Read the model definition and answer for the solid it produces. Units are mm, in the model's axes. A direction names the side the tool comes from. Coordinates: 2 decimals unless noted, no trailing zeros. Write each loop counter-clockwise with the first axis right and the second up, starting at its lowest first coordinate (ties: lowest second). Pieces come first, ordered by that corner, then holes.
(1) Section C-C on z = 3.25 is taken. Write down the section's boundary in (x, y), then the cut area to 3 significant figures.
(2) Which of the six approach directions +Z, -Z, +X, -X, +Y, -Y give full straight-line access (tool end or side, diameter ignored) to faces 4 (the flat face through (2, 0.5, -2)), 5 (the flat face through (7, 0, 10)), 6 (the cylindrical face through (-6.9, 6.95, 10.89))?
(3) The mould has two halves that part along X. Classify faces 1 (the flat face through (-0.598, 4.048, 7.732)), 2 (the cylindrical face through (6.93, 0.25, -4.4)), 3 (the cylindrical face through (-1.952, 0.246, -0.434)): +X half, -X half, draft (parallel to the pull), parting line (faces both ways), or undercut.
(4) Section B-B on z = 0 is taken. Write down the section's boundary in (x, y), then the cut area to 3 significant figures.
(5) Section A-A on x = 0 is taken. Write down the section's boundary in (y, z), then the cut area to 3 significant figures.
(6) Find the intervals of material crossed by probe 1 along X at (y, z) = (0.15, 0); probe 2 along Y at (x, z) = (2, 2.25); probe 3 along X at (y, z) = (4.75, 12.75), in increasing order.
(7) Section D-D on x = 1.5 is taken. Write down the section's boundary in (y, z), then the cut area to 3 significant figures.
(8) Given pin 1 (5 mm diameter, centred on x = -0.5, y = -3, fed in from +Z); pin 2 (6.5 mm diameter, centred on x = 0, z = 0, fed in from -Y); pin 3 (3 mm diameter, centred on x = -4, z = 4, fed in from +Y); pin 4 (7.5 mm diameter, centred on x = -1, z = -0.5, fed in from +Y), each flat-ended and moving along its own axis, determine where each tip first touches the part or whether it passes through.
from build123d import *

# Parameters (mm, degrees)
SKETCH_1_W                       = 15
SKETCH_1_H                       = 10
SKETCH_1_R                       = 2
EXTRUDE_1_DEPTH                  = 0.5
SM_START                         = -7.5
SM_EDGE_FLANGE_1_DEPTH           = 15
SM_EDGE_FLANGE_1_2_DEPTH         = 15
SM_EDGE_FLANGE_2_STRIP_W         = 3
SM_EDGE_FLANGE_2_STRIP_H         = 0.5
SM_EDGE_FLANGE_2_STRIP_CUT_DEPTH = 9.575525184
SM_EDGE_FLANGE_2_DEPTH           = 9.575525184
SKETCH_12_R                      = 1.5
CUT_EXTRUDE_1_DEPTH              = 25.832637406
FILLET_1_R                       = 2


# Read off the part's stored shape, not the designer's step: Ребро-кромка1
# Sheet-metal steps are written as plain solids
with BuildPart() as part:
    # Sketch 1 → Бобышка-Вытянуть1 (new body)
    with BuildSketch(Plane(origin=(0, 0, 0), x_dir=(1, 0, 0), z_dir=(0, 1, 0))):
        Rectangle(SKETCH_1_W, SKETCH_1_H)
        with Locations(Location((0, 0, 0), (0, 0, 270))):
            Circle(SKETCH_1_R, mode=Mode.SUBTRACT)
    extrude(amount=EXTRUDE_1_DEPTH)

    # Ребро-кромка1 outline → Ребро-кромка1 (cut)
    with BuildSketch(Plane.YZ.offset(SM_START)):
        with BuildLine():
            ThreePointArc((0, 4.092680796), (0.079495147, 4.483411925), (0.30534163, 4.812020597))
            Line((0.30534163, 4.812020597), (0.5, 5))
            Line((0.5, 5), (0, 5))
            Line((0, 5), (0, 4.092680796))
        make_face()
    extrude(amount=SM_EDGE_FLANGE_1_DEPTH, mode=Mode.SUBTRACT)

    # Sm Edge Flange 1 2 outline → Sm Edge Flange 1 2 (add)
    with BuildSketch(Plane.YZ.offset(SM_START)):
        with BuildLine():
            Line((7.193398003, 11.463739317), (0.5, 5))
            Line((0.5, 5), (0.5, 4.092680796))
            ThreePointArc((0.5, 4.092680796), (0.539747573, 4.288046361), (0.652670815, 4.452350697))
            Line((0.652670815, 4.452350697), (7.540727189, 11.104069417))
            Line((7.540727189, 11.104069417), (7.193398003, 11.463739317))
        make_face()
    extrude(amount=SM_EDGE_FLANGE_1_2_DEPTH)

    # Ребро-кромка2 strip (across the edge) → Ребро-кромка2 strip cut (cut)
    with BuildSketch(Plane(origin=(7.5, 0.30534163, 4.812020597), x_dir=(-1, 0, 0), z_dir=(0, 0.7193398003386473, 0.6946583704590013))):
        with Locations((-0.5, -0.25)):
            Rectangle(SM_EDGE_FLANGE_2_STRIP_W, SM_EDGE_FLANGE_2_STRIP_H)
    extrude(amount=SM_EDGE_FLANGE_2_STRIP_CUT_DEPTH, mode=Mode.SUBTRACT)

    # Ребро-кромка2 section (across the edge) → Ребро-кромка2 (add)
    with BuildSketch(Plane(origin=(7.5, 0.30534163, 4.812020597), x_dir=(-1, 0, 0), z_dir=(0, 0.7193398003386473, 0.6946583704590013))):
        with BuildLine():
            Line((0, 0.5), (0, 9.5))
            Line((0, 9.5), (0.5, 9.5))
            Line((0.5, 9.5), (0.5, 0.5))
            ThreePointArc((0.5, 0.5), (0.646446609, 0.146446609), (1, 0))
            Line((1, 0), (1, -0.5))
            ThreePointArc((1, -0.5), (0.292893219, -0.207106781), (0, 0.5))
        make_face()
    extrude(amount=SM_EDGE_FLANGE_2_DEPTH)

    # Эскиз12 → Вырез-Вытянуть1 (cut, through all)
    with BuildSketch(Plane(origin=(7.5, 0, 0), x_dir=(0, 0, -1), z_dir=(1, 0, 0))):
        with Locations((-11.879995076, 0.128518841)):
            Circle(SKETCH_12_R)
    extrude(amount=-CUT_EXTRUDE_1_DEPTH, mode=Mode.SUBTRACT)

    # Скругление1
    fillet_1_edges = [part.edges().sort_by_distance(p)[0] for p in [
        (7.25, -6.29391289, 11.6457487),
        (7.25, 0.594143484, 18.29746742),
        (-7.5, 7.367062596, 11.283904367),
        (7.5, 0.25, -5),
        (-7.5, 0.25, -5),
    ]]
    fillet(fillet_1_edges, radius=FILLET_1_R)


solid = part.part
Response:
1. outline: (-7.5, 0) - (7.5, 0) - (7.5, 0.5) - (-7.5, 0.5) - close
1. area: 7.50 mm2
2. face 4: -Z, +X, -X, +Y
2. face 5: +Z, -X, -Y
2. face 6: +Z, -X, +Y
3. face 1: draft
3. face 2: +X half
3. face 3: undercut
4. outline: (-7.5, 0) - (-2, 0) - (-2, 0.5) - (-7.5, 0.5) - close; (2, 0) - (7.5, 0) - (7.5, 0.5) - (2, 0.5) - close
4. area: 5.50 mm2
5. outline: (0, -5) - (0.5, -5) - (0.5, -2) - (0, -2) - close; (0, 2) - (0.5, 2) - (0.5, 4.09) arc R0.5 cw to (0.65, 4.45) - (7.54, 11.1) - (7.19, 11.46) - (0.31, 4.81) arc R1 ccw to (0, 4.09) - close
5. area: 7.64 mm2
6. probe 1: x = -7.5 to -2, 2 to 7.5
6. probe 2: y = 0 to 0.5
6. probe 3: x = 7 to 7.5
7. outline: (0, -5) - (0.5, -5) - (0.5, -1.32) - (0, -1.32) - close; (0, 1.32) - (0.5, 1.32) - (0.5, 4.09) arc R0.5 cw to (0.65, 4.45) - (7.54, 11.1) - (7.19, 11.46) - (0.31, 4.81) arc R1 ccw to (0, 4.09) - close
7. area: 8.31 mm2
8. pin 1: passes through
8. pin 2: stops at y = 0
8. pin 3: stops at y = 1.74
8. pin 4: stops at y = 0.5
